Verification items for the finished model (mm, model axes). A direction names the side the tool comes from. Give positions to 0.01 mm unless a question says otherwise; leave off trailing zeros. Write each loop counter-clockwise with the first axis right and the second up, starting at its lowest first coordinate (ties: lowest second). Pieces come first, ordered by that corner, then holes. Notation, with made-up numbers: (51, 41.25) -> (86, 41.25) arc R26 cw to (86, 59.25) -> close; hole circle Ø9 at (37, -13). An arc over 180 degrees is marked (long way). Use CSV: the item, a comma, the result in double quotes. Start each with the question number.
```python
from build123d import *

# Parameters (mm, degrees)
SKETCH1_W           = 63
SKETCH1_H           = 142
BOSS_EXTRUDE1_DEPTH = 0.75
SKETCH2_W           = 52.632852527
SKETCH2_H           = 10
BOSS_EXTRUDE2_DEPTH = 15
SKETCH3_R           = 6.05981783
SKETCH3_W           = 30.224806401
SKETCH3_H           = 10.769758603
BOSS_EXTRUDE3_DEPTH = 15


with BuildPart() as part:
    # Sketch1 → Boss-Extrude1 (new, symmetric)
    with BuildSketch(Plane.XY):
        Rectangle(SKETCH1_W, SKETCH1_H)
    extrude(amount=BOSS_EXTRUDE1_DEPTH, both=True)

    # Sketch2 → Boss-Extrude2 (add)
    with BuildSketch(Plane.XY.offset(0.75)):
        with Locations((-0.219961356, 60.846409529)):
            Rectangle(SKETCH2_W, SKETCH2_H)
    extrude(amount=BOSS_EXTRUDE2_DEPTH)

    # Sketch3 → Boss-Extrude3 (add)
    with BuildSketch(Plane.XY.offset(0.75)):
        with Locations((17.023166824, -61.057583047)):
            Circle(SKETCH3_R)
        with Locations((-11.11717017, -62.099817751)):
            Rectangle(SKETCH3_W, SKETCH3_H)
    extrude(amount=BOSS_EXTRUDE3_DEPTH)


solid = part.part
```
(1) Set-up check for faces 1 (the face through (-11, -67.485, 8)), 2 (the face through (3.995, -62, 8)), 3 (the face through (-26.536, 61, 8)), 4 (the face through (-11, -56.715, 8)), 5 (the face through (-1, 55.846, 8)): record each of +Z, -Z, +X, -X, +Y, -Y from which the full face is reachable in a straight line by a thin tool's end or side.
(2) Go/stop test with flat-tipped pins: pin 1 (4.5 mm diameter, centred on x = -7, z = 7, fed in from -Y); pin 2 (5.5 mm diameter, centred on y = -62, z = 12, fed in from -X); pin 3 (5 mm diameter, centred on x = 16, y = -9.5, fed in from +Z); pin 4 (1.5 mm diameter, centred on y = 54.5, z = 10.5, fed in from +X). Record where each tip stops, or that it passes through.
(3) Thickness scan on line 1 (Y direction, x = -22, z = 5.5); line 2 (Y direction, x = 17.5, z = 2.75); line 3 (Z direction, x = -4, y = -10.5). Record the ranges inside material, lowest first. Write a range as from..to.
(4) Section check A-A on z = 12. Record the cut outline in (x, y), then the cut area to 3 significant figures.
(5) Draft check along Y on faces 6 (the face through (0, 1, -0.75)), 7 (the face through (0, 1, 0.75)), 8 (the face through (20.281, -55.948, 8.145)), 9 (the face through (-1, 65.846, 8)). Enter one of: released by +Y, released by -Y, zero draft, split by the parting line, or undercut.
(6) Section check C-C on y = 52. Record the cut outline in (x, z), then the cut area to 3 significant figures.
(7) Section check B-B on x = 1. Record the cut outline in (y, z).
(8) Section check D-D on x = 27.5. Record the cut outline in (y, z), then the cut area to 3 significant figures.
Data:
1,face 1,"+Z, +X, -X, -Y"
1,face 2,"+Z, -Y"
1,face 3,"+Z, -X, +Y, -Y"
1,face 4,"+Z, -X"
1,face 5,"+Z, +X, -X"
2,pin 1,"stops at y = -67.48"
2,pin 2,"stops at x = -26.23"
2,pin 3,"stops at z = 0.75"
2,pin 4,"passes through"
3,line 1,"y = -67.48..-56.71, 55.85..65.85"
3,line 2,"y = -67.1..-55.02, 55.85..65.85"
3,line 3,"z = -0.75..0.75"
4,outline,"(-26.54, 55.85) -> (26.1, 55.85) -> (26.1, 65.85) -> (-26.54, 65.85) -> close; (-26.23, -67.48) -> (4, -67.48) -> (4, -56.71) -> (-26.23, -56.71) -> close; circle Ø12.12 at (17.02, -61.06)"
4,area,"967 mm2"
5,face 6,"zero draft"
5,face 7,"undercut"
5,face 8,"undercut"
5,face 9,"released by +Y"
6,outline,"(-31.5, -0.75) -> (31.5, -0.75) -> (31.5, 0.75) -> (-31.5, 0.75) -> close"
6,area,"94.5 mm2"
7,outline,"(-71, -0.75) -> (71, -0.75) -> (71, 0.75) -> (65.85, 0.75) -> (65.85, 15.75) -> (55.85, 15.75) -> (55.85, 0.75) -> (-56.71, 0.75) -> (-56.71, 15.75) -> (-67.48, 15.75) -> (-67.48, 0.75) -> (-71, 0.75) -> close"
8,outline,"(-71, -0.75) -> (71, -0.75) -> (71, 0.75) -> (-71, 0.75) -> close"
8,area,"213 mm2"
